Could you check a few things on this model? Use its own coordinates, in mm. Face numbers are marked on the shaded views. A direction names the side the tool comes from. Give positions to 0.01 mm unless a question says otherwise; leave off trailing zeros. Write each loop counter-clockwise with the first axis right and the second up, starting at its lowest first coordinate (ties: lowest second). Pieces come first, ordered by that corner, then holes. Notation, with made-up numbers: (6, -25.75) - (64, -25.75) arc R30 cw to (64, 9.25) - close; hole circle Ø1 at (8, 78). An arc over 180 degrees is marked (long way). Write item = value, one per line.
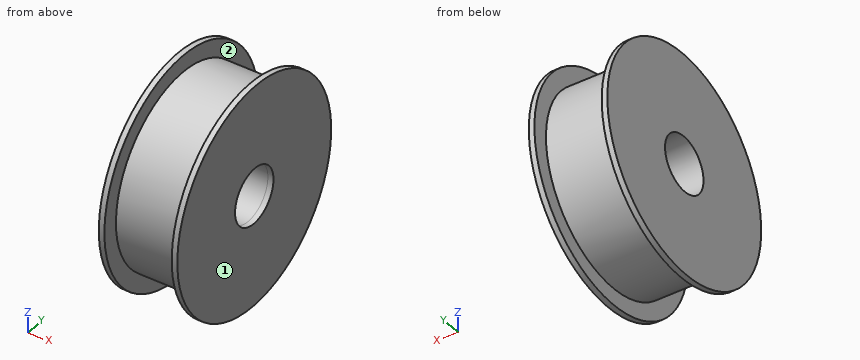
from build123d import *

# Parameters (mm, degrees)
CROQUIS1_R              = 100
CROQUIS1_R_2            = 25
SALIENTE_EXTRUIR1_DEPTH = 5
CROQUIS2_R              = 85
SALIENTE_EXTRUIR2_DEPTH = 60
CROQUIS3_R              = 100
SALIENTE_EXTRUIR3_DEPTH = 5
CROQUIS4_R              = 25
CORTAR_EXTRUIR1_DEPTH   = 65


with BuildPart() as part:
    # Croquis1 → Saliente-Extruir1 (new body)
    with BuildSketch(Plane(origin=(0, 0, 0), x_dir=(0, 0, -1), z_dir=(1, 0, 0))):
        Circle(CROQUIS1_R)
        Circle(CROQUIS1_R_2, mode=Mode.SUBTRACT)
    extrude(amount=SALIENTE_EXTRUIR1_DEPTH)

    # Croquis2 → Saliente-Extruir2 (add)
    with BuildSketch(Plane.ZY):
        Circle(CROQUIS2_R)
    extrude(amount=SALIENTE_EXTRUIR2_DEPTH)

    # Croquis3 → Saliente-Extruir3 (add)
    with BuildSketch(Plane.ZY.offset(60)):
        Circle(CROQUIS3_R)
    extrude(amount=SALIENTE_EXTRUIR3_DEPTH)

    # Croquis4 → Cortar-Extruir1 (cut)
    with BuildSketch(Plane(origin=(0, 0, 0), x_dir=(0, 0, -1), z_dir=(1, 0, 0))):
        Circle(CROQUIS4_R)
    extrude(amount=-CORTAR_EXTRUIR1_DEPTH, mode=Mode.SUBTRACT)


solid = part.part
1. I need wall thicknesses on line 1 (X direction, y = 65, z = 62); line 2 (Y direction, x = 2, z = 0); line 3 (Z direction, x = -21.5, y = -5.5). Which ranges of each line are inside material? Lowest first, please.
Filled sheet:
line_1 = -65 to -60, 0 to 5
line_2 = -100 to -25, 25 to 100
line_3 = -84.82 to -24.39, 24.39 to 84.82
2. If we section it at C-C, the plane x = -6: Please give me the cut outline in (y, z), and give its area (3 significant figures).
Filled sheet:
outline = circle Ø170 at (0, 0); hole circle Ø50 at (0, 0)
area = 20,700 mm2
3. Which directions (+Z, -Z, +X, -X, +Y, -Y) give clear straight access to the entire face, cutting with the end or side of a thin tool? Please do the marked faces 1 and 2.
Filled sheet:
face_1 = +Z, -Z, +X, +Y, -Y
face_2 = none
4. For pin 1 (2 mm diameter, centred on x = -25, y = 50.5, fed in from +Z); pin 2 (5 mm diameter, centred on x = -34, y = 14, fed in from +Z); pin 3 (10 mm diameter, centred on x = -28.5, z = 58.5, fed in from +Y), each with a flat end and sliding along its axis, tell me the tip position at first contact or that it passes through.
Filled sheet:
pin_1 = 69.1
pin_2 = 84.22
pin_3 = 66.05
5. If we section it at A-A, the plane y = 0: Please give me the cut outline in (x, z), and give its area (3 significant figures).
Filled sheet:
outline = (-65, -100) - (-60, -100) - (-60, -85) - (0, -85) - (0, -100) - (5, -100) - (5, -25) - (-65, -25) - close; (-65, 25) - (5, 25) - (5, 100) - (0, 100) - (0, 85) - (-60, 85) - (-60, 100) - (-65, 100) - close
area = 8,700 mm2
6. If we section it at D-D, the plane y = 43.5: Please give me the cut outline in (x, z), and give its area (3 significant figures).
Filled sheet:
outline = (-65, -90.04) - (-60, -90.04) - (-60, -73.03) - (0, -73.03) - (0, -90.04) - (5, -90.04) - (5, 90.04) - (0, 90.04) - (0, 73.03) - (-60, 73.03) - (-60, 90.04) - (-65, 90.04) - close
area = 10,600 mm2
